```python
from build123d import *

# Parameters (mm, degrees)
SKETCH_W        = 12
SKETCH_H        = 12
POCKET_DEPTH    = 6
POCKET001_DEPTH = 3
CHAMFER_SIZE    = 1
CHAMFER001_SIZE = 1


with BuildPart() as part:
    # Sketch002 → Revolution (revolve)
    with BuildSketch(Plane.YZ):
        Polygon((1.6, 13), (1.6, 0), (25, 0), (25, 4), (3, 13), align=None)
    revolve(axis=Axis((0, 0, 0), (0, 0, 1)))

    # Sketch (on Face4 of Revolution) → Pocket (cut)
    with BuildSketch(Plane.YX):
        Rectangle(SKETCH_W, SKETCH_H)
    extrude(amount=-POCKET_DEPTH, mode=Mode.SUBTRACT)

    # Sketch003 (on Face2 of Pocket) → Pocket001 (cut)
    with BuildSketch(Plane.YX.offset(-6)):
        Polygon((3.1, 0), (1.55, 2.684679), (-1.55, 2.684679), (-3.1, 0), (-1.55, -2.684679), (1.55, -2.684679), align=None)
    extrude(amount=-POCKET001_DEPTH, mode=Mode.SUBTRACT)

    # Chamfer
    chamfer_edges = [part.edges().sort_by_distance(p)[0] for p in [
        (0, -6, 6),
        (0, 6, 6),
        (-6, 0, 6),
        (6, 0, 6),
    ]]
    chamfer(chamfer_edges, length=CHAMFER_SIZE)

    # Chamfer001
    chamfer001_edges = [part.edges().sort_by_distance(p)[0] for p in [
        (0, -1.6, 9),
    ]]
    chamfer(chamfer001_edges, length=CHAMFER001_SIZE)


solid = part.part
```
CAD build for the part. Positions are in the model's coordinates, mm. A direction names the side the tool comes from. Coordinates: 2 decimals unless noted, no trailing zeros. Order: outer loops, then holes, each group sorted by start corner. A loop starts at its lowest first (then second) coordinate and runs counter-clockwise, first axis right, second up. Notation, with made-up numbers: M 74.5,20 L 126.5,20 A18 cw 126.5,27 Z; hole C -4,61 d11. An arc over 180 degrees is marked long. Answer as CSV lines item,"result".
1) Drill centre lines: L1, parallel to Y at x = 0, z = 11.1; L2, parallel to X at y = 2, z = 0.75; L3, parallel to Y at x = 0, z = 11.4. Where is each one in solid material? Low to high. Write a range as from..to.
Verdict:
L1,"-7.64..-1.6, 1.6..7.64"
L2,"-24.92..-6, 6..24.92"
L3,"-6.91..-1.6, 1.6..6.91"
2) Cut at C-C (z = 8). List the corners of the cut face in (x, y), then the cut area to 3 significant figures.
Verdict:
outline,"C 0,0 d30.44; hole M -2.68,-1.55 L 0,-3.1 L 2.68,-1.55 L 2.68,1.55 L 0,3.1 L -2.68,1.55 Z"
area,"703 mm2"
3) Cut at A-A (y = 0). List the corners of the cut face in (x, z).
Verdict:
outline,"M -25,0 L -6,0 L -6,5 L -5,6 L -2.68,6 L -2.68,9 L -2.6,9 L -1.6,10 L -1.6,13 L -3,13 L -25,4 Z; M 1.6,10 L 2.6,9 L 2.68,9 L 2.68,6 L 5,6 L 6,5 L 6,0 L 25,0 L 25,4 L 3,13 L 1.6,13 Z"
4) Cut at B-B (z = 2.5). List the corners of the cut face in (x, y), then the cut area to 3 significant figures.
Verdict:
outline,"C 0,0 d50; hole M -6,-6 L 6,-6 L 6,6 L -6,6 Z"
area,"1,820 mm2"
5) 3-axis set-ups, long thin cutter, end or side, ignore diameter. For faces 4 (the conical face through (-4.034, -0.53, 12.563)), 5 (the flat face through (-2.685, 0, 7)): which of +Z, -Z, +X, -X, +Y, -Y reach the whole face in a straight line?
Verdict:
face 4,"+Z"
face 5,"-Z"
6) Flat gauge pins, fed straight in: P1, Ø4.5, axis at x = 1, y = 1, coming from the -Z side; P2, Ø5, axis at x = 16, y = 15, coming from the +Z side; P3, Ø0.9, axis at y = 0.5, z = 8, coming from the -X side. Where does each tip first touch, or does it go through?
Verdict:
P1,"z = 6"
P2,"z = 6.28"
P3,"x = -16.31"
7) Mould opens along X. For faces 1 (the flat face through (1.3, 1.3, 13)), 2 (the cylindrical face through (-7.509, 23.846, 2.028)), 3 (the flat face through (-6, 0, 2)) say: released by +X, released by -X, zero draft, split by the parting line, or undercut.
Verdict:
face 1,"zero draft"
face 2,"split by the parting line"
face 3,"undercut"
